Answer from the drawing. Dimensions are ordinates in mm from the lowest x, y and z of the part. Round coordinates to 2 decimals unless told otherwise and drop trailing zeros. Loops run counter-clockwise (first coordinate to the right, second up) from the corner with the lowest first, then second, coordinate; pieces in that order, holes last. Notation, with made-up numbers: (-22.75, -9) - (19.25, -9) arc R13 ccw to (19.25, 5) - close; hole circle Ø4 at (-5.75, -39.75). An arc over 180 degrees is marked (long way). Return JSON: item names as keys, results as strings.
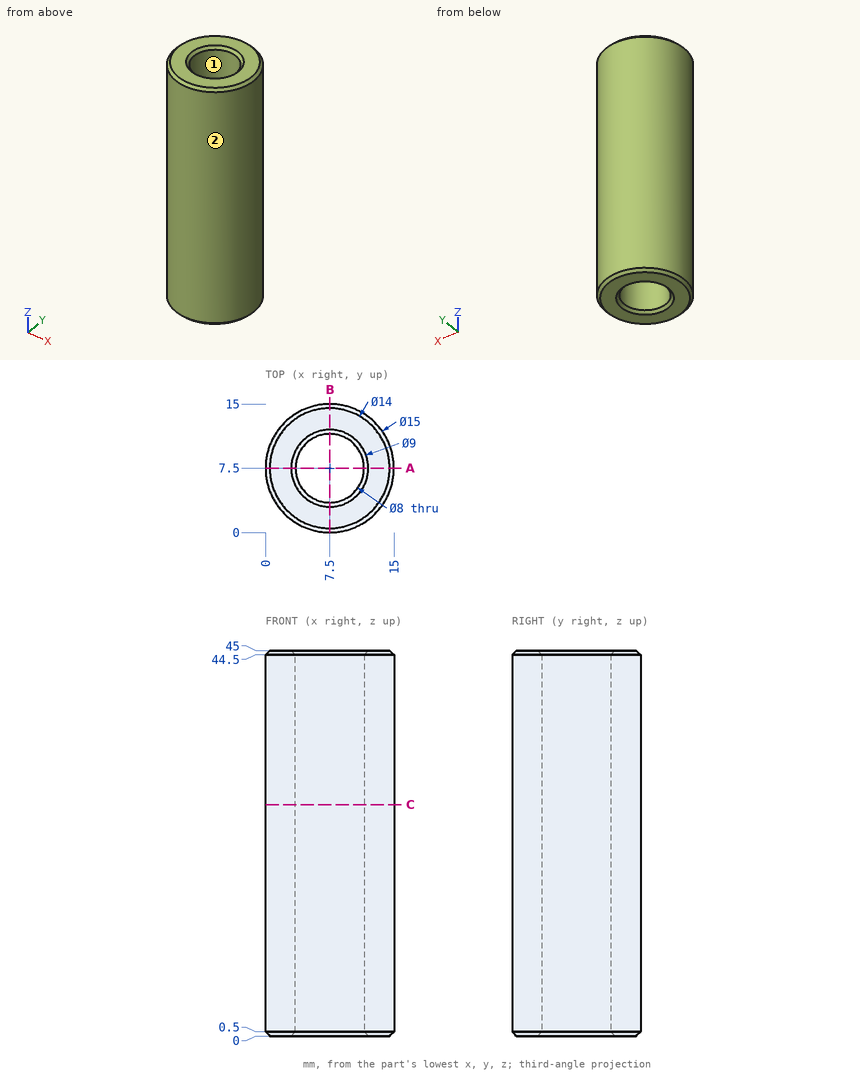
1) Section C-C (z = 27) is taken. Give the vertices of the cut face in (x, y).
Verdict:
{"outline": "circle Ø15 at (7.5, 7.5); hole circle Ø8 at (7.5, 7.5)"}
2) Flat-ended cylindrical pins translate along their axes: pin 1 (1 mm diameter, centred on x = 2, z = 9, fed in from -Y); pin 2 (6 mm diameter, centred on x = 5.5, z = 27.5, fed in from +Y); pin 3 (1.5 mm diameter, centred on x = 12.5, z = 7, fed in from -Y); pin 4 (1.5 mm diameter, centred on y = 10.5, z = 16, fed in from -X). Find the tip coordinate at first contact, or state that the pin passes through.
Verdict:
{"pin 1": "stops at y = 1.91", "pin 2": "stops at y = 15", "pin 3": "stops at y = 1.32", "pin 4": "stops at x = 0.35"}
3) Determine the mould class of the marked faces 1 and 2 for opening direction X: pulls with the +X half, pulls with the -X half, needs draft (parallel to the pull), parting line crosses it, or undercut.
Verdict:
{"face 1": "undercut", "face 2": "parting line crosses it"}
4) Section A-A (y = 7.5) is taken. Give the vertices of the cut face in (x, z), and give its area (3 significant figures).
Verdict:
{"outline": "(0, 0.5) - (0.5, 0) - (3, 0) - (3.5, 0.5) - (3.5, 44.5) - (3, 45) - (0.5, 45) - (0, 44.5) - close; (11.5, 0.5) - (12, 0) - (14.5, 0) - (15, 0.5) - (15, 44.5) - (14.5, 45) - (12, 45) - (11.5, 44.5) - close", "area": "314 mm2"}
5) Find the intervals of material crossed by L1, parallel to Y at x = 7.5, z = 24; L2, parallel to X at y = 7.75, z = 23; L3, parallel to Y at x = 6.5, z = 3, in increasing order.
Verdict:
{"L1": "y = 0 to 3.5, 11.5 to 15", "L2": "x = 0 to 3.51, 11.49 to 15", "L3": "y = 0.07 to 3.63, 11.37 to 14.93"}
